from build123d import *
from build123d.topology import SkipClean

# Parameters (mm, degrees)
SKETCH1_R           = 7.9375
BOSS_EXTRUDE1_DEPTH = 6.35
BOSS_EXTRUDE1_DRAFT = -1
CUT_EXTRUDE3_DEPTH  = 8.9375
CIRPATTERN3_COUNT   = 9
SKETCH7_R           = 7.9375
SKETCH7_R_2         = 5.5245
BOSS_EXTRUDE3_DEPTH = 6.35
BOSS_EXTRUDE3_DRAFT = -1
DRAFT1_ANGLE        = -10
FILLET2_R           = 0.508


with BuildPart() as part:
    # Sketch1 → Boss-Extrude1 (with draft: the straight prism first)
    with BuildSketch(Plane(origin=(0, 0, 0), x_dir=(1, 0, 0), z_dir=(0, 1, 0))):
        Circle(SKETCH1_R)
    extrude(amount=-BOSS_EXTRUDE1_DEPTH)
    # Boss-Extrude1: the draft: its side faces are tilted about the plane it starts from
    boss_extrude1_sides = [part.faces().sort_by_distance(p)[0] for p in [
        (-7.9375, -3.175, 0),
    ]]
    draft(boss_extrude1_sides, Plane(origin=(0, 0, 0), x_dir=(1, 0, 0), z_dir=(0, 1, 0)), BOSS_EXTRUDE1_DRAFT)

    # Sketch6 → Cut-Extrude3 (cut, through all)
    with BuildSketch(Plane.XY):
        Polygon((0, -2.413), (-7.112, -9.525), (7.112, -9.525), align=None)
    cut_extrude3 = extrude(amount=-CUT_EXTRUDE3_DEPTH, mode=Mode.SUBTRACT)

    # CirPattern3: Cut-Extrude3 ×9 about axis
    cirpattern3_axis = Axis((0, 0, 0), (0, 1, 0))
    for i in range(1, CIRPATTERN3_COUNT):
        add(cut_extrude3.rotate(cirpattern3_axis, i * 360 / CIRPATTERN3_COUNT), mode=Mode.SUBTRACT)


with BuildPart() as boss_extrude3_tool:
    # Sketch7 → Boss-Extrude3 (with draft: the straight prism first)
    with BuildSketch(Plane(origin=(0, 0, 0), x_dir=(1, 0, 0), z_dir=(0, 1, 0))):
        Circle(SKETCH7_R)
        Circle(SKETCH7_R_2, mode=Mode.SUBTRACT)
    extrude(amount=-BOSS_EXTRUDE3_DEPTH)
    # Boss-Extrude3: the draft: its side faces are tilted about the plane it starts from
    boss_extrude3_sides = [boss_extrude3_tool.faces().sort_by_distance(p)[0] for p in [
        (-7.9375, -3.175, 0),
        (-5.5245, -3.175, 0),
    ]]
    draft(boss_extrude3_sides, Plane(origin=(0, 0, 0), x_dir=(1, 0, 0), z_dir=(0, 1, 0)), BOSS_EXTRUDE3_DRAFT)


with BuildPart() as part_1:
    add(part.part)

    # Boss-Extrude3: add boss_extrude3_tool
    add(boss_extrude3_tool.part)

    # Draft1
    draft1_faces = [part_1.faces().sort_by_distance(p)[0] for p in [
        (-5.600979367, -4.381499996, 0),
    ]]
    draft(draft1_faces, Plane.ZX, DRAFT1_ANGLE)

    # Fillet2
    fillet2_edges = [part_1.edges().sort_by_distance(p)[0] for p in [
        (-7.826660338, -6.35, 0),
        (-6.644176327, -6.35, 0),
    ]]
    fillet(fillet2_edges, radius=FILLET2_R)

    # Sketch8 → Cut-Revolve1 (revolve, cut)
    with SkipClean():  # keep this step's faces unmerged: merging them makes the solid invalid here
        with BuildSketch(Plane(origin=(0, 0, 0), x_dir=(0, 0, -1), z_dir=(1, 0, 0))):
            with BuildLine():
                Line((-5.800063528, -2.413), (-5.800063528, -6.720189325))
                Line((-5.800063528, -6.720189325), (-6.570156602, -6.720189325))
                Line((-6.570156602, -6.720189325), (-6.570156602, -5.930213274))
                Line((-6.570156602, -5.930213274), (-5.949977004, -2.413))
                ThreePointArc((-5.949977004, -2.413), (-5.875020266, -2.350103828), (-5.800063528, -2.413))
            make_face()
        revolve(axis=Axis((0, 0, 0), (0, -1, 0)), mode=Mode.SUBTRACT)


solid = part_1.part
Can you work these out from the model? Positions are in its coordinate system, mm. A direction names the side the tool comes from. Coordinates: 2 decimals unless noted, no trailing zeros. Write each loop counter-clockwise with the first axis right and the second up, starting at its lowest first coordinate (ties: lowest second). Pieces come first, ordered by that corner, then holes. Notation, with made-up numbers: (68.25, 6.25) - (108.25, 6.25) arc R33 ccw to (108.25, 37.25) - close; hole circle Ø11 at (31.25, 46). An arc over 180 degrees is marked (long way). Return JSON: item names as keys, results as strings. Group by question number.
Item 1: If we section it at C-C (y = -5): Write out the boundary of the cut face in (x, z), then the cut area to 3 significant figures.
Item 2: Please list where these lines run through material, in increasing order: probe 1 along Z at (x, y) = (4.25, -3.75); probe 2 along X at (y, z) = (-1.25, 6); probe 3 along Z at (x, y) = (2.5, -4.5).
Item 3: If we section it at A-A (y = -3.75): Count the separate pieces of the cut face and the enclosed holes in it, then the cut area to 3 significant figures.
Item 4: Which directions (+Z, -Z, +X, -X, +Y, -Y) give clear straight access to the entire face, cutting with the end or side of a thin tool? Please do faces 1 (the face through (0, 0, 0)), 2 (the face through (3.2, -3.198, 2.754)).
Item 5: I'm going to push flat-ended pins straight in: pin 1 Ø1.5 at (x, z) = (-2.5, -3) entering from -Y; pin 2 Ø3 at (y, z) = (-5, 5.5) entering from +X; pin 3 Ø1.5 at (x, z) = (-6, 5.5) entering from -Y. Where does each tip first touch, or does it pass through?
Return value:
{
 "1": {"outline": "circle Ø15.7 at (0, 0); hole circle Ø12.81 at (0, 0)", "area": "64.7 mm^2"},
 "2": {"probe 1": "z = -6.63 to -4.49, -2.98 to -2.11, 0.61 to 0.91, 4.49 to 6.63", "probe 2": "x = -5.16 to 5.16", "probe 3": "z = -7.45 to -5.8, 5.8 to 7.45"},
 "3": {"separate pieces": "10", "enclosed holes": "1", "area": "86.0 mm^2"},
 "4": {"face 1": "+Z, -Z, +X, -X, +Y", "face 2": "-Y"},
 "5": {"pin 1": "stops at y = -3.18", "pin 2": "stops at x = 6.76", "pin 3": "stops at y = -6.35"}
}
